CAD build for the part. Positions are in the model's coordinates, mm. A direction names the side the tool comes from. Give positions to 0.01 mm unless a question says otherwise; leave off trailing zeros. Put each result on its own line as item: value. Start each with the question number.
1. Wall check: line 1 (Y direction, x = -15, z = 8); line 2 (X direction, y = -28, z = 1.75); line 3 (Y direction, x = -47.5, z = 2). Give the ranges that are in metal, low to high.
2. Mould opens along Y. For faces 4 (the flat face through (-1.934, -39.263, 9.86)), 5 (the cylindrical face through (5.82, 54.19, 9.86)), 6 (the flat face through (-43.84, 8.61, 9.86)) say: +Y half, -Y half, draft (parallel to the pull), parting line (faces both ways), or undercut.
3. Drop flat-ended pins along their axis: pin 1 (1 mm diameter, centred on x = -26, y = -42.5, fed in from -Z); pin 2 (8 mm diameter, centred on y = -14, z = 12.5, fed in from +X); pin 3 (8 mm diameter, centred on x = 5.5, z = 4, fed in from +Y); pin 4 (8 mm diameter, centred on x = -3, z = 4.5, fed in from -Y). Give the stop position or say it passes through.
4. Tool access for faces 1 (the flat face through (-16.094, -41.679, 9.86)), 2 (the flat face through (-21.06, -31.07, 10.04)), 3 (the cylindrical face through (38.165, 35.917, 9.86)): list every direction of +Z, -Z, +X, -X, +Y, -Y with a clear straight run to the whole face (end or side of a thin tool).
5. Cut at A-A on z = 1.75. Give the number of separate pieces and of enclosed holes in the cut face, and give its area (3 significant figures).
from build123d import *

# Parameters (mm, degrees)
F0_R      = 22.5
F1_DEPTH  = 20
F2_R      = 2.5
F3_DEPTH  = 20.001
F4_R      = 2.5
F5_DEPTH  = 5
F6_R      = 2.5
F7_DEPTH  = 5
F8_R      = 2.5
F9_DEPTH  = 5
F10_R     = 2.5
F11_DEPTH = 5
F12_R     = 2.5
F13_DEPTH = 5
F14_R     = 2.5
F15_DEPTH = 5
F16_R     = 2.5
F17_DEPTH = 5
F18_R     = 2.5
F19_DEPTH = 5
F20_R     = 2.5
F21_DEPTH = 5


# Not quite as in the source:
# - a feature names something its author has since deleted; it is built from what else it names


with BuildPart() as f1:
    # F0 (on Top) → F1 (new body)
    with BuildSketch(Plane.XY):
        with BuildLine():
            ThreePointArc((50, 2.2360679775), (52.3585771958, 2.9784933095), (54.4735576923, 1.6975017946))
            ThreePointArc((54.4735576923, 1.6975017946), (54.3740921627, 3.7024453378), (54.2008581475, 5.7023658309))
            Line((54.2008581475, 5.7023658309), (33.7982304406, 8.1353188741))
            Line((33.7982304406, 8.1353188741), (36.8649053656, 33.8523079329))
            ThreePointArc((36.8649053656, 33.8523079329), (38.1944585155, 35.9371029308), (40.6380330461, 36.3152897571))
            ThreePointArc((40.6380330461, 36.3152897571), (39.2730851622, 37.7872304071), (37.8548560942, 39.207905709))
            Line((37.8548560942, 39.207905709), (20.6616644432, 27.9570995731))
            Line((20.6616644432, 27.9570995731), (6.4803118028, 49.62867678))
            ThreePointArc((6.4803118028, 49.62867678), (6.1587282118, 52.0803426945), (7.7875210962, 53.9407500428))
            ThreePointArc((7.7875210962, 53.9407500428), (5.7957651426, 54.1909504107), (3.7961461645, 54.3676307585))
            Line((3.7961461645, 54.3676307585), (-2.1427239761, 34.6974426733))
            Line((-2.1427239761, 34.6974426733), (-26.9364916731, 42.1832362005))
            ThreePointArc((-26.9364916731, 42.1832362005), (-28.7587394689, 43.8546113028), (-28.7068585233, 46.3267338987))
            ThreePointArc((-28.7068585233, 46.3267338987), (-30.3934578, 45.2381224517), (-32.038822745, 44.0881371472))
            Line((-32.038822745, 44.0881371472), (-23.9445080332, 25.2024667275))
            Line((-23.9445080332, 25.2024667275), (-47.7494113294, 14.9997905883))
            ThreePointArc((-47.7494113294, 14.9997905883), (-50.2196733343, 15.1088198928), (-51.7689799985, 17.0359240992))
            ThreePointArc((-51.7689799985, 17.0359240992), (-52.3612440523, 15.1178742319), (-52.8824704203, 13.1793141796))
            Line((-52.8824704203, 13.1793141796), (-34.542390668, 3.9149765057))
            Line((-34.542390668, 3.9149765057), (-46.2198507491, -19.2022237443))
            ThreePointArc((-46.2198507491, -19.2022237443), (-48.1822639171, -20.7065562608), (-50.6078203843, -20.2261839196))
            ThreePointArc((-50.6078203843, -20.2261839196), (-49.8286222822, -22.0761953575), (-48.9818224627, -23.8962563644))
            Line((-48.9818224627, -23.8962563644), (-28.9775048134, -19.2043747332))
            Line((-28.9775048134, -19.2043747332), (-23.0635083269, -44.419304178))
            ThreePointArc((-23.0635083269, -44.419304178), (-23.5998377269, -46.8331046123), (-25.766699169, -48.0242356934))
            ThreePointArc((-25.766699169, -48.0242356934), (-23.9806343627, -48.9405677895), (-22.1620354025, -49.7905029782))
            Line((-22.1620354025, -49.7905029782), (-9.8537224074, -33.3377856016))
            Line((-9.8537224074, -33.3377856016), (10.8845059639, -48.8520985212))
            ThreePointArc((10.8845059639, -48.8520985212), (12.0252148188, -51.0459228237), (11.1309469524, -53.3512138563))
            ThreePointArc((11.1309469524, -53.3512138563), (13.0881588901, -52.905104639), (15.0276143261, -52.3872198887))
            Line((15.0276143261, -52.3872198887), (13.8807262249, -31.8720760788))
            Line((13.8807262249, -31.8720760788), (39.7395389463, -30.4264530357))
            ThreePointArc((39.7395389463, -30.4264530357), (42.0235357053, -31.3737864336), (42.8202992881, -33.7145661232))
            ThreePointArc((42.8202992881, -33.7145661232), (44.0328571396, -32.1147550532), (45.1856762982, -30.4713743942))
            Line((45.1856762982, -30.4713743942), (31.1202287894, -15.49306794))
            Line((31.1202287894, -15.49306794), (50, 2.2360679775))
        make_face()
        Circle(F0_R, mode=Mode.SUBTRACT)
    extrude(amount=F1_DEPTH)

    # F2 (on face) → F3 (cut, through all)
    with BuildSketch(Plane.XY.offset(20)):
        with Locations((15, 25.9807621135)):
            Circle(F2_R)
        with BuildLine():
            ThreePointArc((32.5, 0), (30, 2.5), (27.5, 0))
            ThreePointArc((27.5, 0), (30, -2.5), (32.5, 0))
        make_face()
        with Locations((15, -25.9807621135)):
            Circle(F2_R)
        with Locations((-15, -25.9807621135)):
            Circle(F2_R)
        with Locations((-30, 0)):
            Circle(F2_R)
        with Locations((-15, 25.9807621135)):
            Circle(F2_R)
    extrude(amount=-F3_DEPTH, mode=Mode.SUBTRACT)

    # F4 (on face) → F5 (cut)
    with BuildSketch(Plane(origin=(32.3678514777, -3.8597706083, 0), x_dir=(0.1184081423, 0.9929650104, 0), z_dir=(0.9929650104, -0.1184081423, 0))):
        with Locations((25.4792622567, 10)):
            Circle(F4_R)
    extrude(amount=-F5_DEPTH, mode=Mode.SUBTRACT)

    # F6 (on face) → F7 (cut)
    with BuildSketch(Plane(origin=(27.2762254834, 17.8488980559, 0), x_dir=(-0.5475597061, 0.8367666151, 0), z_dir=(0.8367666151, 0.5475597061, 0))):
        with Locations((25.4792622567, 10)):
            Circle(F6_R)
    extrude(amount=-F7_DEPTH, mode=Mode.SUBTRACT)

    # F8 (on face) → F9 (cut)
    with BuildSketch(Plane(origin=(9.421750444, 31.2058689513, 0), x_dir=(-0.9573182826, 0.289035821, 0), z_dir=(0.289035821, 0.9573182826, 0))):
        with Locations((25.4792622567, 10)):
            Circle(F8_R)
    extrude(amount=-F9_DEPTH, mode=Mode.SUBTRACT)

    # F10 (on face) → F11 (cut)
    with BuildSketch(Plane(origin=(-12.8412663393, 29.9612669498, 0), x_dir=(-0.9191369952, -0.393938046, 0), z_dir=(-0.393938046, 0.9191369952, 0))):
        with Locations((25.4792622567, 10)):
            Circle(F10_R)
    extrude(amount=-F11_DEPTH, mode=Mode.SUBTRACT)

    # F12 (on face) → F13 (cut)
    with BuildSketch(Plane(origin=(-29.0957118877, 14.6974551601, 0), x_dir=(-0.4508812927, -0.8925839232, 0), z_dir=(-0.8925839232, 0.4508812927, 0))):
        with Locations((25.4792622567, 10)):
            Circle(F12_R)
    extrude(amount=-F13_DEPTH, mode=Mode.SUBTRACT)

    # F14 (on face) → F15 (cut)
    with BuildSketch(Plane(origin=(-31.735950481, -7.4434592431, 0), x_dir=(0.2283467777, -0.9735798627, 0), z_dir=(-0.9735798627, -0.2283467777, 0))):
        with Locations((25.4792622567, 10)):
            Circle(F14_R)
    extrude(amount=-F15_DEPTH, mode=Mode.SUBTRACT)

    # F16 (on face) → F17 (cut)
    with BuildSketch(Plane(origin=(-19.5265851384, -26.1014963415, 0), x_dir=(0.8007288529, -0.5990269644, 0), z_dir=(-0.5990269644, -0.8007288529, 0))):
        with Locations((25.4792622567, 10)):
            Circle(F16_R)
    extrude(amount=-F17_DEPTH, mode=Mode.SUBTRACT)

    # F18 (on face) → F19 (cut)
    with BuildSketch(Plane(origin=(1.8194864043, -32.546353216, 0), x_dir=(0.9984409988, 0.055817308, 0), z_dir=(0.055817308, -0.9984409988, 0))):
        with Locations((25.4792622567, 10)):
            Circle(F18_R)
    extrude(amount=-F19_DEPTH, mode=Mode.SUBTRACT)

    # F20 (on face) → F21 (cut)
    with BuildSketch(Plane(origin=(22.314200037, -23.7624097082, 0), x_dir=(0.7289715049, 0.6845440417, 0), z_dir=(0.6845440417, -0.7289715049, 0))):
        with Locations((25.4792622567, 10)):
            Circle(F20_R)
    extrude(amount=-F21_DEPTH, mode=Mode.SUBTRACT)


solid = f1.part
Report:
1. line 1: y = -40.22 to -28.48, -23.48 to -16.77, 16.77 to 23.48, 28.48 to 33.36
1. line 2: x = -26.91 to -16.47, -13.53 to 13.53, 16.47 to 42.86
1. line 3: y = -23.55 to -20.46, 10.46 to 15.11
2. face 4: -Y half
2. face 5: +Y half
2. face 6: undercut
3. pin 1: passes through
3. pin 2: stops at x = 36.97
3. pin 3: stops at y = 54.37
3. pin 4: stops at y = -41.46
4. face 1: +Z, -Z, -Y
4. face 2: none
4. face 3: +Z, -Z
5. separate pieces: 1
5. enclosed holes: 7
5. area: 4,000 mm²
